Model file for the job. Use its own axes, mm. Coordinates: 2 decimals unless noted, no trailing zeros. Write each loop counter-clockwise with the first axis right and the second up, starting at its lowest first coordinate (ties: lowest second). Pieces come first, ordered by that corner, then holes.
Q1. Pin check, flat tips, straight feed: P1, Ø4, axis at x = -6.5, y = -6, coming from the -Z side; P2, Ø10, axis at y = -6.5, z = 57.5, coming from the +X side; P3, Ø5, axis at y = -6.5, z = 9, coming from the +X side; P4, Ø1.5, axis at x = 5.5, z = 22.5, coming from the +Y side. Stop position of each tip, or through.
Q2. Band-saw the part on A-A, the plane z = 54.5. Write the cut outline in (x, y).
Q3. Drill centre lines: probe 1 along Y at (x, z) = (0.5, 62.5); probe 2 along Y at (x, z) = (-4.75, 7). Where is each one in solid material? Low to high.
from build123d import *

# Parameters (mm, degrees)
F0_R     = 9
F1_DEPTH = 65
F2_R     = 1.5
F3_R     = 1.5
F5_R     = 1


with BuildPart() as f1:
    # F0 (on Top) → F1 (new body)
    with BuildSketch(Plane.XY):
        Circle(F0_R)
    extrude(amount=F1_DEPTH)

    # F2
    f2_edges = [f1.edges().sort_by_distance(p)[0] for p in [
        (-9, 0, 65),
        (-9, 0, 0),
    ]]
    fillet(f2_edges, radius=F2_R)

    # F3 (on Front) → F4 (revolve, cut)
    with BuildSketch(Plane.XZ):
        with Locations((10.25, 61)):
            Circle(F3_R)
    revolve(axis=Axis((0, 0, 65), (0, 0, 1)), mode=Mode.SUBTRACT)

    # F5
    f5_edges = [f1.edges().sort_by_distance(p)[0] for p in [
        (-9, 0, 60.170844),
        (-9, 0, 61.829156),
    ]]
    fillet(f5_edges, radius=F5_R)


solid = f1.part
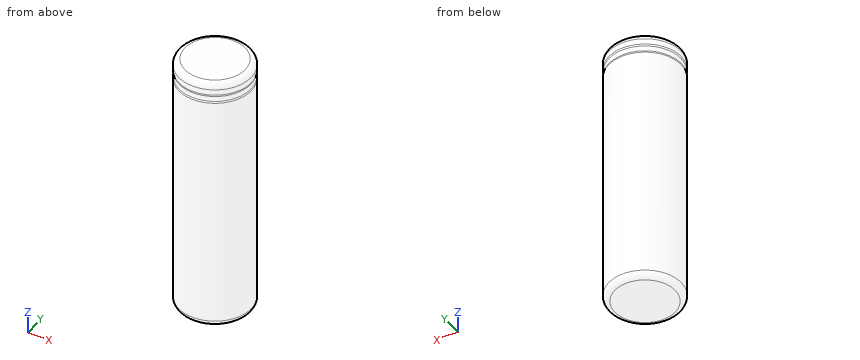
Answer sheet:
1. P1: stops at z = 0
1. P2: stops at x = 8.87
1. P3: stops at x = 8.06
1. P4: stops at y = 7.64
2. outline: circle Ø18 at (0, 0)
3. probe 1: y = -8.99 to 8.99
3. probe 2: y = -7.64 to 7.64
